Check sheet for the modelled part. Datum: model origin and axes. Units: mm. A direction names the side the tool comes from. Give positions to 0.01 mm unless a question says otherwise; leave off trailing zeros. Write each loop counter-clockwise with the first axis right and the second up, starting at its lowest first coordinate (ties: lowest second). Pieces come first, ordered by that corner, then holes. Notation, with made-up numbers: M 65,43 L 92,43 A27 cw 92,60 Z; hole C 14.5,46.5 d1. An arc over 180 degrees is marked long. Write item = value, one per line. Start each with the question number.
1) Access from +Z, -Z, +X, -X, +Y, -Y to the whole of each face (thin tool, end or side, straight path). Record for faces 5 (the flat face through (12, 1, 40)), 6 (the flat face through (20, 5, -50)), 7 (the flat face through (19.1, 5.58, -15.72)), 8 (the flat face through (-20, 5, -52)).
2) Scan lines: line 1 along X through (y, z) = (4.25, 40); line 2 along Z through (x, y) = (13, 4); line 3 along X through (y, z) = (2.75, -35). Record each from-to range of solid material in increasing order. Write a range as [from, to].
3) Cross-section at C-C, the plane z = 35. Record the cut outline in (x, y), plus the area to 3 significant figures.
4) Cross-section at B-B, the plane x = -24. Record the cut outline in (y, z).
5) Mould release check, pull along Z, two halves, no side actions. Record for faces 1 (the flat face through (-24, 0, -13)), 2 (the flat face through (-35, 5, 50)), 3 (the flat face through (-12.72, 5.58, -16.1)), 4 (the flat face through (18.72, 5.58, 16.1)): released by +Z, released by -Z, zero draft, split by the parting line, or undercut.
6) Cross-section at D-D, the plane x = 12. Record the cut outline in (y, z), plus the area to 3 significant figures.
7) Go/stop test with flat-tipped pins: pin 1 (1.5 mm diameter, centred on x = 22.5, y = 2.5, fed in from +Z); pin 2 (1.5 mm diameter, centred on y = 6.5, z = 53.5, fed in from +X); pin 3 (5.5 mm diameter, centred on x = -31.5, y = 6, fed in from -Z). Record where each tip stops, or that it passes through.
8) Cross-section at A-A, the plane y = 3. Record the cut outline in (x, z).
```python
from build123d import *

# Parameters (mm, degrees)
SKETCH1_R           = 4
BOSS_EXTRUDE1_DEPTH = 11
SKETCH2_R           = 1.5
CUT_EXTRUDE1_DEPTH  = 10
CUT_EXTRUDE2_DEPTH  = 11
FILLET1_R           = 3


with BuildPart() as part:
    # Sketch1 → Boss-Extrude1 (new body)
    with BuildSketch(Plane(origin=(0, 0, 0), x_dir=(1, 0, 0), z_dir=(0, 1, 0))):
        Polygon((0, 50), (40, 50), (40, -50), (0, -50), (0, -55), (-20, -55), (-20, -50), (-40, -50), (-50, -50), (-50, 50), (-40, 50), (-20, 50), (-20, 55), (0, 55), align=None)
        with Locations(Location((-35, 35, 0), (0, 0, 270))):
            Circle(SKETCH1_R, mode=Mode.SUBTRACT)
        with Locations(Location((-35, -35, 0), (0, 0, 90))):
            Circle(SKETCH1_R, mode=Mode.SUBTRACT)
    extrude(amount=BOSS_EXTRUDE1_DEPTH)

    # Sketch2 → Cut-Extrude1 (cut)
    with BuildSketch(Plane(origin=(0, 11, 0), x_dir=(1, 0, 0), z_dir=(0, 1, 0))):
        with Locations(Location((32, -40, 0), (0, 0, 270))):
            Circle(SKETCH2_R)
        with Locations(Location((12, -40, 0), (0, 0, 90))):
            Circle(SKETCH2_R)
    extrude(amount=-CUT_EXTRUDE1_DEPTH, mode=Mode.SUBTRACT)

    # Sketch3 → Cut-Extrude2 (cut)
    with BuildSketch(Plane(origin=(0, 11, 0), x_dir=(1, 0, 0), z_dir=(0, 1, 0))):
        Polygon((-28.819805153, 0), (3, -31.819805153), (34.819805153, 0), (3, 31.819805153), align=None)
    extrude(amount=-CUT_EXTRUDE2_DEPTH, mode=Mode.SUBTRACT)

    # Fillet1
    fillet1_edges = [part.edges().sort_by_distance(p)[0] for p in [
        (-28.819805153, 5.5, 0),
        (3, 5.5, -31.819805153),
        (34.819805153, 5.5, 0),
        (3, 5.5, 31.819805153),
    ]]
    fillet(fillet1_edges, radius=FILLET1_R)


solid = part.part
```
Reply:
q1.face_5 = +Y
q1.face_6 = -Z, +X, +Y, -Y
q1.face_7 = +Y, -Y
q1.face_8 = -Z, -X, +Y, -Y
q2.line_1 = [-50, 10.5], [13.5, 30.5], [33.5, 40]
q2.line_2 = [-50, -21.82], [21.82, 38.88], [41.12, 50]
q2.line_3 = [-50, -39], [-31, 40]
q3.outline = M -50,0 L -39,0 L -39,11 L -50,11 Z; M -31,0 L 40,0 L 40,11 L -31,11 Z
q3.area = 902 mm2
q4.outline = M 0,-50 L 11,-50 L 11,-4.82 L 0,-4.82 Z; M 0,4.82 L 11,4.82 L 11,50 L 0,50 Z
q5.face_1 = zero draft
q5.face_2 = released by +Z
q5.face_3 = undercut
q5.face_4 = undercut
q6.outline = M 0,-50 L 11,-50 L 11,-22.82 L 0,-22.82 Z; M 0,22.82 L 11,22.82 L 11,38.5 L 1,38.5 L 1,41.5 L 11,41.5 L 11,50 L 0,50 Z
q6.area = 568 mm2
q7.pin_1 = 50
q7.pin_2 = 0
q7.pin_3 = -50
q8.outline = M -50,-50 L -20,-50 L -20,-55 L 0,-55 L 0,-50 L 40,-50 L 40,50 L 0,50 L 0,55 L -20,55 L -20,50 L -50,50 Z; hole C -35,-35 d8; hole C -35,35 d8; hole M -26.7,-2.12 L 0.88,-29.7 A3 ccw 5.12,-29.7 L 32.7,-2.12 A3 ccw 32.7,2.12 L 5.12,29.7 A3 ccw 0.88,29.7 L -26.7,2.12 A3 ccw Z; hole C 12,40 d3; hole C 32,40 d3
